from build123d import *
from build123d.topology import SkipClean

# Parameters (mm, degrees)
SKETCH_1_R          = 2.5
EXTRUDE_228_DEPTH   = 10
EXTRUDE_1_DEPTH     = 1.5
EXTRUDE_2_DEPTH     = 3
SKETCH_4_R          = 6
EXTRUDE_3_DEPTH     = 1.5
SKETCH_5_R          = 3
EXTRUDE_4_DEPTH     = 10
CHAMFER_1_SIZE      = 0.5
SKETCH_6_R          = 2.5
CUT_EXTRUDE_2_DEPTH = 1.5


with BuildPart() as part:
    # Эскиз1 → Extrude 228 (new body)
    with BuildSketch(Plane.XY):
        Circle(SKETCH_1_R)
    extrude(amount=EXTRUDE_228_DEPTH)

    # Эскиз2 → Бобышка-Вытянуть1 (add)
    with BuildSketch(Plane.XY.offset(10)):
        with BuildLine():
            Line((-3, 2.645751311), (-3, -2.645751311))
            ThreePointArc((-3, -2.645751311), (0, -4), (3, -2.645751311))
            Line((3, -2.645751311), (3, 2.645751311))
            ThreePointArc((3, 2.645751311), (0, 4), (-3, 2.645751311))
        make_face()
    extrude(amount=EXTRUDE_1_DEPTH)

    # Эскиз3 → Бобышка-Вытянуть2 (add)
    with BuildSketch(Plane.XY.offset(11.5)):
        Polygon((0, -6.92820323), (6, -3.464101615), (6, 3.464101615), (0, 6.92820323), (-6, 3.464101615), (-6, -3.464101615), align=None)
    extrude(amount=EXTRUDE_2_DEPTH)

    # Эскиз4 → Бобышка-Вытянуть3 (add)
    with BuildSketch(Plane.XY.offset(14.5)):
        Circle(SKETCH_4_R)
    extrude(amount=EXTRUDE_3_DEPTH)

    # Эскиз5 → Бобышка-Вытянуть4 (add)
    with BuildSketch(Plane.XY.offset(16)):
        Circle(SKETCH_5_R)
    extrude(amount=EXTRUDE_4_DEPTH)

    # Фаска1
    chamfer_1_edges = [part.edges().sort_by_distance(p)[0] for p in [
        (-2.5, 0, 0),
        (-3, 0, 26),
    ]]
    chamfer(chamfer_1_edges, length=CHAMFER_1_SIZE)

    # Эскиз6 → Вырез-Вытянуть2 (cut)
    with SkipClean():  # the faces are left unmerged after this step: merging them gives an invalid solid
        with BuildSketch(Plane(origin=(0, 0, 10), x_dir=(-1, 0, 0), z_dir=(0, 0, -1))):
            with BuildLine():
                Line((-3, 2.645751311), (-3, -2.645751311))
                ThreePointArc((-3, -2.645751311), (0, -4), (3, -2.645751311))
                Line((3, -2.645751311), (3, 2.645751311))
                ThreePointArc((3, 2.645751311), (0, 4), (-3, 2.645751311))
            make_face()
            Circle(SKETCH_6_R, mode=Mode.SUBTRACT)
        extrude(amount=-CUT_EXTRUDE_2_DEPTH, mode=Mode.SUBTRACT)


solid = part.part
Verification items for the finished model (mm, model axes). A direction names the side the tool comes from. Give positions to 0.01 mm unless a question says otherwise; leave off trailing zeros. Loops run counter-clockwise (first coordinate to the right, second up) from the corner with the lowest first, then second, coordinate; pieces in that order, holes last.
1) Sectioned sample at C-C, the plane z = 18.5. Enter the section's corners in (x, y), then the cut area to 3 significant figures.
2) Sectioned sample at B-B, the plane y = -4.5. Enter the section's corners in (x, z).
3) Sectioned sample at A-A, the plane z = 13.25. Enter the section's corners in (x, y).
4) Depth check by flat-ended pin: pin 1 Ø1.5 at (x, z) = (1.5, 9) entering from -Y; pin 2 Ø0.9 at (x, y) = (-5, -3.5) entering from +Z; pin 3 Ø1 at (x, z) = (-0.5, 7.5) entering from +Y. Enter the tip coordinate at first touch or a pass-through.
5) Sectioned sample at D-D, the plane z = 4. Enter the section's corners in (x, y).
6) Thickness scan on line 1 along Y through (x, z) = (0, 4.75); line 2 along Z through (x, y) = (5, 3); line 3 along Y through (x, z) = (-3, 12.75). Record the ranges inside material, lowest first.
7) Draft check along Z on faces 6 (the flat face through (0, -6.2, 14.5)), 7 (the flat face through (-6, 0, 13)), 8 (the flat face through (0, 0, 0)). Enter one of: pulls with the +Z half, pulls with the -Z half, needs draft (parallel to the pull), parting line crosses it, or undercut.
8) Set-up check for faces 1 (the flat face through (-3, -1, 16)), 2 (the flat face through (-5.4, -3.2, 14.5)), 3 (the flat face through (5.4, 3, 14.5)), 4 (the flat face through (-5.4, 3, 14.5)), 5 (the flat face through (-2.96, 5.22, 12.98)): record each of +Z, -Z, +X, -X, +Y, -Y from which the full face is reachable in a straight line by a thin tool's end or side.
Answers:
1. outline: circle Ø6 at (0, 0)
1. area: 28.3 mm2
2. outline: (-4.21, 11.5) - (4.21, 11.5) - (4.21, 14.5) - (3.97, 14.5) - (3.97, 16) - (-3.97, 16) - (-3.97, 14.5) - (-4.21, 14.5) - close
3. outline: (-6, -3.46) - (0, -6.93) - (6, -3.46) - (6, 3.46) - (0, 6.93) - (-6, 3.46) - close
4. pin 1: stops at y = -2.38
4. pin 2: stops at z = 16
4. pin 3: stops at y = 2.5
5. outline: circle Ø5 at (0, 0)
6. line 1: y = -2.5 to 2.5
6. line 2: z = 11.5 to 16
6. line 3: y = -5.2 to 5.2
7. face 6: pulls with the +Z half
7. face 7: needs draft
7. face 8: pulls with the -Z half
8. face 1: +Z
8. face 2: +Z, -X, -Y
8. face 3: +Z, +X, +Y
8. face 4: +Z, -X, +Y
8. face 5: +Z, -Z, -X, +Y
